Build history of the part. All positions in model axes, mm. A direction names the side the tool comes from. Round coordinates to 2 decimals unless told otherwise and drop trailing zeros. Loops run counter-clockwise (first coordinate to the right, second up) from the corner with the lowest first, then second, coordinate; pieces in that order, holes last.
from build123d import *

# Parameters (mm, degrees)
SKETCH1_W           = 70
SKETCH1_H           = 25.5
SKETCH1_R           = 1.7
SKETCH1_W_2         = 12
SKETCH1_H_2         = 12
BOSS_EXTRUDE1_DEPTH = 10
SKETCH1_3_W         = 12
SKETCH1_3_H         = 12
SKETCH1_3_R         = 5
BOSS_EXTRUDE2_DEPTH = 5


with BuildPart() as part:
    # Sketch1 → Boss-Extrude1 (new body)
    with BuildSketch(Plane(origin=(0, 0, 0), x_dir=(1, 0, 0), z_dir=(0, 1, 0))):
        Rectangle(SKETCH1_W, SKETCH1_H)
        with Locations((29.875, 0)):
            Circle(SKETCH1_R, mode=Mode.SUBTRACT)
        with Locations((-29.625, 0)):
            Circle(SKETCH1_R, mode=Mode.SUBTRACT)
        with Locations((3.25, 6.25)):
            Rectangle(SKETCH1_W_2, SKETCH1_H_2, mode=Mode.SUBTRACT)
        with Locations((-3.75, -6.25)):
            Rectangle(SKETCH1_W_2, SKETCH1_H_2, mode=Mode.SUBTRACT)
        with Locations((-17.75, -6.25)):
            Rectangle(SKETCH1_W_2, SKETCH1_H_2, mode=Mode.SUBTRACT)
        with Locations((10.75, -6.25)):
            Rectangle(SKETCH1_W_2, SKETCH1_H_2, mode=Mode.SUBTRACT)
        with Locations((18.25, 6.25)):
            Rectangle(SKETCH1_W_2, SKETCH1_H_2, mode=Mode.SUBTRACT)
        with Locations((-10.75, 6.25)):
            Rectangle(SKETCH1_W_2, SKETCH1_H_2, mode=Mode.SUBTRACT)
    extrude(amount=-BOSS_EXTRUDE1_DEPTH)

    # Sketch1_3 → Boss-Extrude2 (add)
    with BuildSketch(Plane(origin=(0, 0, 0), x_dir=(1, 0, 0), z_dir=(0, 1, 0))):
        with Locations((-10.75, 6.25)):
            Rectangle(SKETCH1_3_W, SKETCH1_3_H)
        with Locations((-10.75, 6.25)):
            Circle(SKETCH1_3_R, mode=Mode.SUBTRACT)
        with Locations((3.25, 6.25)):
            Rectangle(SKETCH1_3_W, SKETCH1_3_H)
        with Locations((3.394505145, 6.25)):
            Circle(SKETCH1_3_R, mode=Mode.SUBTRACT)
        with Locations((18.25, 6.25)):
            Rectangle(SKETCH1_3_W, SKETCH1_3_H)
        with Locations((18.25, 6.25)):
            Circle(SKETCH1_3_R, mode=Mode.SUBTRACT)
        with Locations((10.75, -6.25)):
            Rectangle(SKETCH1_3_W, SKETCH1_3_H)
        with Locations((10.75, -6.25)):
            Circle(SKETCH1_3_R, mode=Mode.SUBTRACT)
        with Locations((-3.75, -6.25)):
            Rectangle(SKETCH1_3_W, SKETCH1_3_H)
        with Locations((-3.75, -6.25)):
            Circle(SKETCH1_3_R, mode=Mode.SUBTRACT)
        with Locations((-17.75, -6.25)):
            Rectangle(SKETCH1_3_W, SKETCH1_3_H)
        with Locations((-17.75, -6.25)):
            Circle(SKETCH1_3_R, mode=Mode.SUBTRACT)
    extrude(amount=-BOSS_EXTRUDE2_DEPTH)


solid = part.part
(1) Slice it at A-A on y = -1.5. Count the separate pieces of the cut face and the enclosed holes in it, plus the area to 3 significant figures.
Responses:
separate pieces: 1
enclosed holes: 8
area: 1,300 mm2
(2) Which spindle directions (+Z, -Z, +X, -X, +Y, -Y) get a long thin tool onto all of the face, cutting with end or side? Do faces 4 (the face through (-28.055, -4.93, 0.651)), 5 (the face through (12.25, -7, -6)). Say none if no direction does.
Responses:
face 4: +Y, -Y
face 5: -Y
(3) Slice it at C-C on z = -8. List the corners of the cut face in (x, y).
Responses:
outline: (-35, -10) - (-16.75, -10) - (-16.75, -5) - (-15.43, -5) - (-15.43, 0) - (-35, 0) - close; (-6.07, -5) - (-4.75, -5) - (-4.75, -10) - (-2.75, -10) - (-2.75, -5) - (-1.29, -5) - (-1.29, 0) - (-6.07, 0) - close; (8.08, -5) - (9.25, -5) - (9.25, -10) - (12.25, -10) - (12.25, -5) - (13.57, -5) - (13.57, 0) - (8.08, 0) - close; (22.93, -5) - (24.25, -5) - (24.25, -10) - (35, -10) - (35, 0) - (22.93, 0) - close
(4) Slice it at D-D on x = 7. List the corners of the cut face in (y, z), plus the area to 3 significant figures.
Responses:
outline: (-10, -12.75) - (0, -12.75) - (0, -9.71) - (-5, -9.71) - (-5, -12.25) - (-10, -12.25) - close; (-10, -0.25) - (-5, -0.25) - (-5, -2.79) - (0, -2.79) - (0, 2.94) - (-5, 2.94) - (-5, 0.25) - (-10, 0.25) - close; (-10, 12.25) - (-5, 12.25) - (-5, 9.56) - (0, 9.56) - (0, 12.75) - (-10, 12.75) - close
area: 67.3 mm2
(5) Pin check, flat tip, straight feed: P1, Ø1, axis at x = -14.5, z = 1, coming from the -Y side. Stop position of the tip, or through.
Responses:
P1: stops at y = -5
(6) Probe line 1 (X direction, y = -3.5, z = 6.25); line 2 (X direction, y = -2.2, z = -6.25); line 3 (X direction, y = -5.75, z = 0) (3 decimals). List the from-to ranges inside material, lowest first.
Responses:
line 1: x = -35 to -22.75, -12.75 to -8.75, 1.25 to 5.75, 15.75 to 35
line 2: x = -35 to -15.75, -5.75 to -1.61, 8.39 to 13.25, 23.25 to 35
line 3: x = -35 to -31.325, -27.925 to 28.175, 31.575 to 35
(7) Slice it at B-B on x = -10.75. List the corners of the cut face in (y, z), plus the area to 3 significant figures.
Responses:
outline: (-10, -12.75) - (0, -12.75) - (0, -11.25) - (-5, -11.25) - (-5, -12.25) - (-10, -12.25) - close; (-10, -0.25) - (-5, -0.25) - (-5, -1.25) - (0, -1.25) - (0, 12.75) - (-10, 12.75) - close
area: 145 mm2
(8) Pull direction Z, two halves, no side cores. Call faces 1 (the face through (-2.75, -7, -6)), 2 (the face through (0, -5, 12.75)), 3 (the face through (-35, -5, 0)): +Z half, -Z half, draft (parallel to the pull), parting line (faces both ways), or undercut.
Responses:
face 1: undercut
face 2: +Z half
face 3: draft
